Here's how the part is built. I have some questions about the finished solid (model axes, mm). A direction names the side the tool comes from. Coordinates: 2 decimals unless noted, no trailing zeros. Write each loop counter-clockwise with the first axis right and the second up, starting at its lowest first coordinate (ties: lowest second). Pieces come first, ordered by that corner, then holes.
Item 1: If we mould it in two halves opening along Y, with no side actions, what happens to faces 1 (the face through (0, 8, 15.875)), 2 (the face through (-14.985, 0.66, 0.298)), 3 (the face through (-0.13, -6.76, 10.56)), 4 (the face through (-0.13, 8.74, 10.56))? For each: pulls with the +Y half, pulls with the -Y half, needs draft (parallel to the pull), parting line crosses it, or undercut.
Item 2: For faces 5 (the face through (-9, 11, -5.125)), 6 (the face through (0, 0, -5.875)), which set-ups out of +Z, -Z, +X, -X, +Y, -Y let a thin tool reach every point of the face, with its end or its side?
Item 3: Please list where these lines run through material, in increasing order: line 1 (Z direction, x = -4, y = -5) (3 decimals); line 2 (Z direction, x = 4.5, y = 12.5) (3 decimals); line 3 (Y direction, x = 9.5, z = -3.5).
Item 4: I'm going to push flat-ended pins straight in: P1, Ø2, axis at x = 1, y = 0.5, coming from the +Z side (3 decimals); P2, Ø10, axis at y = -11.5, z = 4.5, coming from the +X side; P3, Ø6, axis at y = -11.5, z = 5, coming from the +X side; P4, Ø10, axis at x = 8.5, z = 13.5, coming from the +Y side. Where does each tip first touch, or does it pass through?
Item 5: I want a section at A-A (z = 11.5). Please give me the cut outline in (x, y), and give its area (3 significant figures).
from build123d import *

# Parameters (mm, degrees)
FILLET1_R           = 10
SKETCH3_R           = 1
BOSS_EXTRUDE1_DEPTH = 10
FILLET2_R           = 0.5


with BuildPart() as part:
    # Sketch2 → Revolve1 (revolve)
    with BuildSketch(Plane(origin=(0, 0, 0), x_dir=(1, 0, 0), z_dir=(0, 1, 0))):
        with BuildLine():
            Line((0, -5.875), (15, -5.875))
            Line((15, -5.875), (15, 5.125))
            Line((15, 5.125), (12.5, 5.125))
            add(Edge.make_bspline(
                [(12.5, 5.125), (9.5, 5.875)],
                knots=[0, 0, 1, 1], degree=1))
            Line((9.5, 5.875), (0, 5.875))
            Line((0, 5.875), (0, -5.875))
        make_face()
    revolve(axis=Axis((0, 0, 0), (0, 0, 1)))

    # Fillet1
    fillet1_edges = [part.edges().sort_by_distance(p)[0] for p in [
        (-12.5, 0, -5.125),
        (-9.5, 0, -5.875),
    ]]
    fillet(fillet1_edges, radius=FILLET1_R)

    # Sketch3 → Boss-Extrude1 (add)
    with BuildSketch(Plane.XY.offset(5.875)):
        with Locations((0, 7.75)):
            Circle(SKETCH3_R)
        with Locations((0, -7.75)):
            Circle(SKETCH3_R)
    extrude(amount=BOSS_EXTRUDE1_DEPTH)

    # Fillet2
    fillet2_edges = [part.edges().sort_by_distance(p)[0] for p in [
        (-1, 7.75, 15.875),
        (-1, -7.75, 15.875),
    ]]
    fillet(fillet2_edges, radius=FILLET2_R)


solid = part.part
Answer:
1. face 1: needs draft
1. face 2: parting line crosses it
1. face 3: undercut
1. face 4: undercut
2. face 5: -Z
2. face 6: -Z, +X, -X, +Y, -Y
3. line 1: z = -5.875 to 5.875
3. line 2: z = -5.135 to 5.875
3. line 3: y = -11.61 to 11.61
4. P1: stops at z = 5.875
4. P2: stops at x = 13.52
4. P3: stops at x = 12.36
4. P4: passes through
5. outline: circle Ø2 at (0, -7.75); circle Ø2 at (0, 7.75)
5. area: 6.28 mm2
